The listing builds one solid part. Answer for the finished solid, in the listing's coordinates (mm). Coordinates: 2 decimals unless noted, no trailing zeros. Loops run counter-clockwise (first coordinate to the right, second up) from the corner with the lowest first, then second, coordinate; pieces in that order, holes last. Notation, with made-up numbers: (-34, 86) - (-12, 86) arc R15 cw to (-12, 114) - close; hole circle Ø1 at (31, 37). An arc over 180 degrees is marked (long way). Put each result on its own line as item: value.
```python
from build123d import *

# Parameters (mm, degrees)
SKETCH1_W           = 1220
SKETCH1_H           = 102
BOSS_EXTRUDE1_DEPTH = 12
SKETCH4_W           = 84.308730764
SKETCH4_H           = 36.280116476
SKETCH4_W_2         = 1001.25
SKETCH4_H_2         = 42.963295827
SKETCH4_W_3         = 112.735688249
CUT_EXTRUDE1_DEPTH  = 20
SKETCH5_W           = 107.106738726
SKETCH5_H           = 164.152719134
SKETCH5_W_2         = 109.43514609
SKETCH5_H_2         = 176.958959634
CUT_EXTRUDE2_DEPTH  = 20
SKETCH6_R           = 2.5
CUT_EXTRUDE3_DEPTH  = 20
SKETCH7_R           = 2.5
CUT_EXTRUDE4_DEPTH  = 22
SKETCH8_W           = 20.5
SKETCH8_H           = 12.1
CUT_EXTRUDE5_DEPTH  = 20
SKETCH9_R           = 3
CUT_EXTRUDE6_DEPTH  = 20


with BuildPart() as part:
    # Sketch1 → Boss-Extrude1 (new body)
    with BuildSketch(Plane(origin=(0, 0, 0), x_dir=(0, 0, -1), z_dir=(1, 0, 0))):
        with Locations((610, 51)):
            Rectangle(SKETCH1_W, SKETCH1_H)
    extrude(amount=BOSS_EXTRUDE1_DEPTH)

    # Sketch4 → Cut-Extrude1 (cut)
    with BuildSketch(Plane(origin=(12, 0, 0), x_dir=(0, 0, -1), z_dir=(1, 0, 0))):
        with Locations((27.220634618, -6.140058238)):
            Rectangle(SKETCH4_W, SKETCH4_H)
        with Locations((610, -9.481647914)):
            Rectangle(SKETCH4_W_2, SKETCH4_H_2)
        with Locations((1206.992844125, -9.481647914)):
            Rectangle(SKETCH4_W_3, SKETCH4_H_2)
    extrude(amount=-CUT_EXTRUDE1_DEPTH, mode=Mode.SUBTRACT)

    # Sketch5 → Cut-Extrude2 (cut)
    with BuildSketch(Plane(origin=(12, 0, 0), x_dir=(0, 0, -1), z_dir=(1, 0, 0))):
        with Locations((1263.553369363, 24.432676068)):
            Rectangle(SKETCH5_W, SKETCH5_H)
        with Locations((-44.717573045, 30.835796318)):
            Rectangle(SKETCH5_W_2, SKETCH5_H_2)
    extrude(amount=-CUT_EXTRUDE2_DEPTH, mode=Mode.SUBTRACT)

    # Sketch6 → Cut-Extrude3 (cut)
    with BuildSketch(Plane(origin=(12, 0, 0), x_dir=(0, 0, -1), z_dir=(1, 0, 0))):
        with Locations((89.375, 95)):
            Circle(SKETCH6_R)
        with Locations((238.125, 95)):
            Circle(SKETCH6_R)
        with Locations((386.875, 95)):
            Circle(SKETCH6_R)
        with Locations((535.625, 95)):
            Circle(SKETCH6_R)
        with Locations((684.375, 95)):
            Circle(SKETCH6_R)
        with Locations((833.125, 95)):
            Circle(SKETCH6_R)
        with Locations((981.875, 95)):
            Circle(SKETCH6_R)
        with Locations((1130.625, 95)):
            Circle(SKETCH6_R)
    extrude(amount=-CUT_EXTRUDE3_DEPTH, mode=Mode.SUBTRACT)

    # Sketch7 → Cut-Extrude4 (cut)
    with BuildSketch(Plane(origin=(12, 0, 0), x_dir=(0, 0, -1), z_dir=(1, 0, 0))):
        with Locations((99.375, 85)):
            Circle(SKETCH7_R)
        with Locations((248.125, 85)):
            Circle(SKETCH7_R)
        with Locations((396.875, 85)):
            Circle(SKETCH7_R)
        with Locations((545.625, 85)):
            Circle(SKETCH7_R)
        with Locations((694.375, 85)):
            Circle(SKETCH7_R)
        with Locations((843.125, 85)):
            Circle(SKETCH7_R)
        with Locations((991.875, 85)):
            Circle(SKETCH7_R)
        with Locations((1140.625, 85)):
            Circle(SKETCH7_R)
    extrude(amount=-CUT_EXTRUDE4_DEPTH, mode=Mode.SUBTRACT)

    # Sketch8 → Cut-Extrude5 (cut)
    with BuildSketch(Plane(origin=(12, 0, 0), x_dir=(0, 0, -1), z_dir=(1, 0, 0))):
        with Locations((89.625, 18.05)):
            Rectangle(SKETCH8_W, SKETCH8_H)
        with Locations((1130.875, 18.05)):
            Rectangle(SKETCH8_W, SKETCH8_H)
    extrude(amount=-CUT_EXTRUDE5_DEPTH, mode=Mode.SUBTRACT)

    # Sketch9 → Cut-Extrude6 (cut)
    with BuildSketch(Plane(origin=(12, 0, 0), x_dir=(0, 0, -1), z_dir=(1, 0, 0))):
        with Locations((40, 18)):
            Circle(SKETCH9_R)
        with Locations((325, 18)):
            Circle(SKETCH9_R)
        with Locations((610, 18)):
            Circle(SKETCH9_R)
        with Locations((895, 18)):
            Circle(SKETCH9_R)
        with Locations((1180, 18)):
            Circle(SKETCH9_R)
    extrude(amount=-CUT_EXTRUDE6_DEPTH, mode=Mode.SUBTRACT)


solid = part.part
```
1) The part is cut by section A-A (z = -927). Give the vertices of the cut face in (x, y).
Found:
outline: (0, 12) - (12, 12) - (12, 102) - (0, 102) - close
2) Each of these flat-tipped pins is pushed along its axis until it touches: pin 1 (5.5 mm diameter, centred on y = 18, z = -1180, fed in from +X); pin 2 (3.5 mm diameter, centred on x = 5.5, y = 7, fed in from -Z) (3 decimals); pin 3 (6 mm diameter, centred on x = 2, z = -781.5, fed in from -Y). Where does it stop, or does it pass through?
Found:
pin 1: passes through
pin 2: stops at z = -1150.625
pin 3: stops at y = 12
3) Straight lines are drawn through the part: L1, parallel to Y at x = 3.5, z = -325; L2, parallel to Y at x = 7.5, z = -262.5; L3, parallel to Z at x = 5.5, y = 7 (3 decimals). For each, find the intervals that lie inside material, in ascending order. Write a range as [from, to].
Found:
L1: y = [12, 15], [21, 102]
L2: y = [12, 102]
L3: z = [-1150.625, -1110.625], [-109.375, -69.375]
4) The part is cut by section B-B (x = 5). State how many separate pieces and enclosed holes the cut face has, and give its area (3 significant figures).
Found:
separate pieces: 1
enclosed holes: 23
area: 108,000 mm^2
